Answer from the drawing. Dimensions are ordinates in mm from the lowest x, y and z of the part. Round coordinates to 2 decimals unless told otherwise and drop trailing zeros. Write each loop counter-clockwise with the first axis right and the second up, starting at its lowest first coordinate (ties: lowest second). Pieces come first, ordered by that corner, then holes. Notation, with made-up numbers: (76, 13) - (93, 13) arc R37 cw to (93, 52) - close; hole circle Ø10 at (-12, 11.25). An arc over 180 degrees is marked (long way). Answer as CSV lines item,"result". Start each with the question number.
1) Find section C-C on y = 4.75. Determine the outline of the cut face in (x, z), then the cut area to 3 significant figures.
2) Find section A-A on z = 7. Determine the outline of the cut face in (x, y).
3) Find section B-B on x = 2.5. Determine the outline of the cut face in (y, z), then the cut area to 3 significant figures.
4) Consider line 1 along Z through (x, y) = (3.5, 2.75); line 2 along X through (y, z) = (6, 6.5); line 3 along Y through (x, z) = (3.25, 7.75). Determine where each line is inside the solid, lowest interval first.
5) This flat-tipped pin is pushed along its axis until it touches: pin 1 (1.5 mm diameter, centred on y = 2.5, z = 2.5, fed in from +X). Where does it stop, or does it pass through?
6) For a pull along X with two mould halves and no side action, classify the marked faces 1, 2 and 3 as +X half, -X half, draft (parallel to the pull), parting line (faces both ways), or undercut.
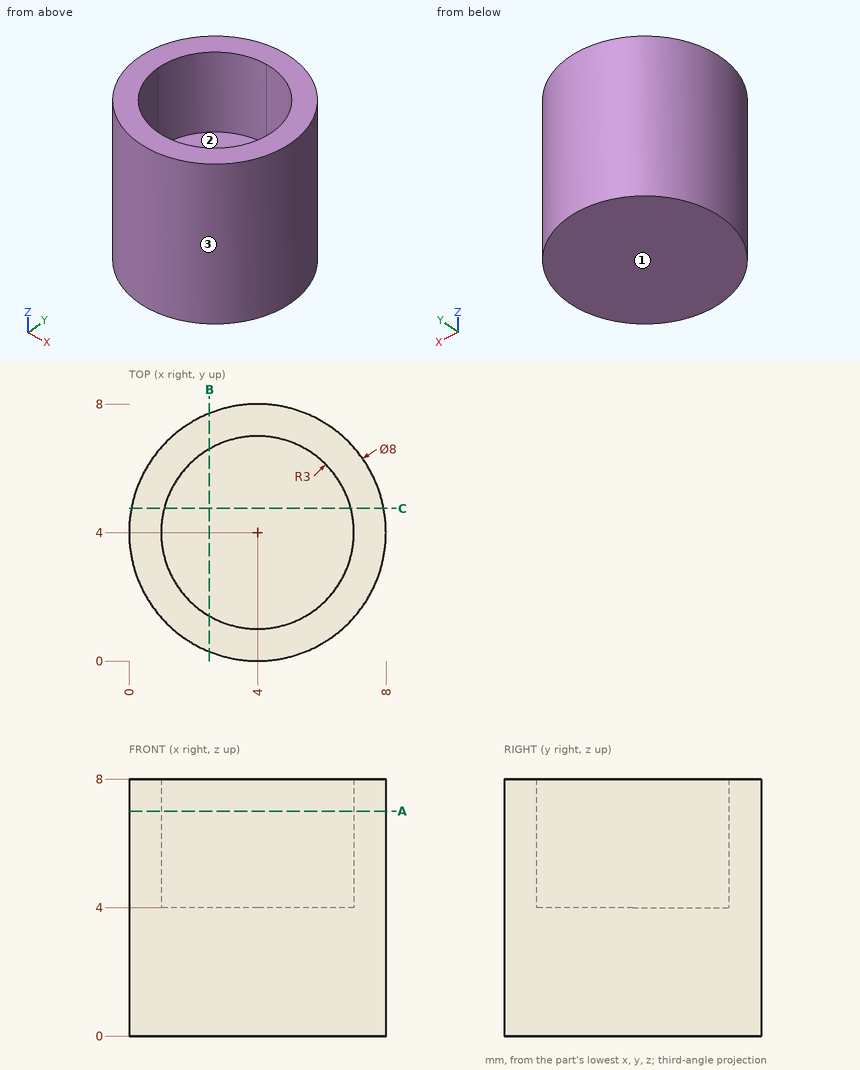
Check values:
1,outline,"(0.07, 0) - (7.93, 0) - (7.93, 8) - (6.9, 8) - (6.9, 4) - (1.1, 4) - (1.1, 8) - (0.07, 8) - close"
1,area,"39.6 mm^2"
2,outline,"circle Ø8 at (4, 4); hole (1, 4) arc R3 ccw to (4, 1) arc R3 ccw to (7, 4) arc R3 ccw to (4, 7) arc R3 ccw to start"
3,outline,"(0.29, 0) - (7.71, 0) - (7.71, 8) - (6.6, 8) - (6.6, 4) - (1.4, 4) - (1.4, 8) - (0.29, 8) - close"
3,area,"38.5 mm^2"
4,line 1,"z = 0 to 4"
4,line 2,"x = 0.54 to 1.76, 6.24 to 7.46"
4,line 3,"y = 0.07 to 1.1, 6.9 to 7.93"
5,pin 1,"stops at x = 7.93"
6,face 1,"draft"
6,face 2,"undercut"
6,face 3,"parting line"
